Can you work these out from the drawing? Everything is in mm from the part's minimum corner. Coordinates: 2 decimals unless noted, no trailing zeros. Loops run counter-clockwise (first coordinate to the right, second up) from the corner with the lowest first, then second, coordinate; pieces in that order, holes last.
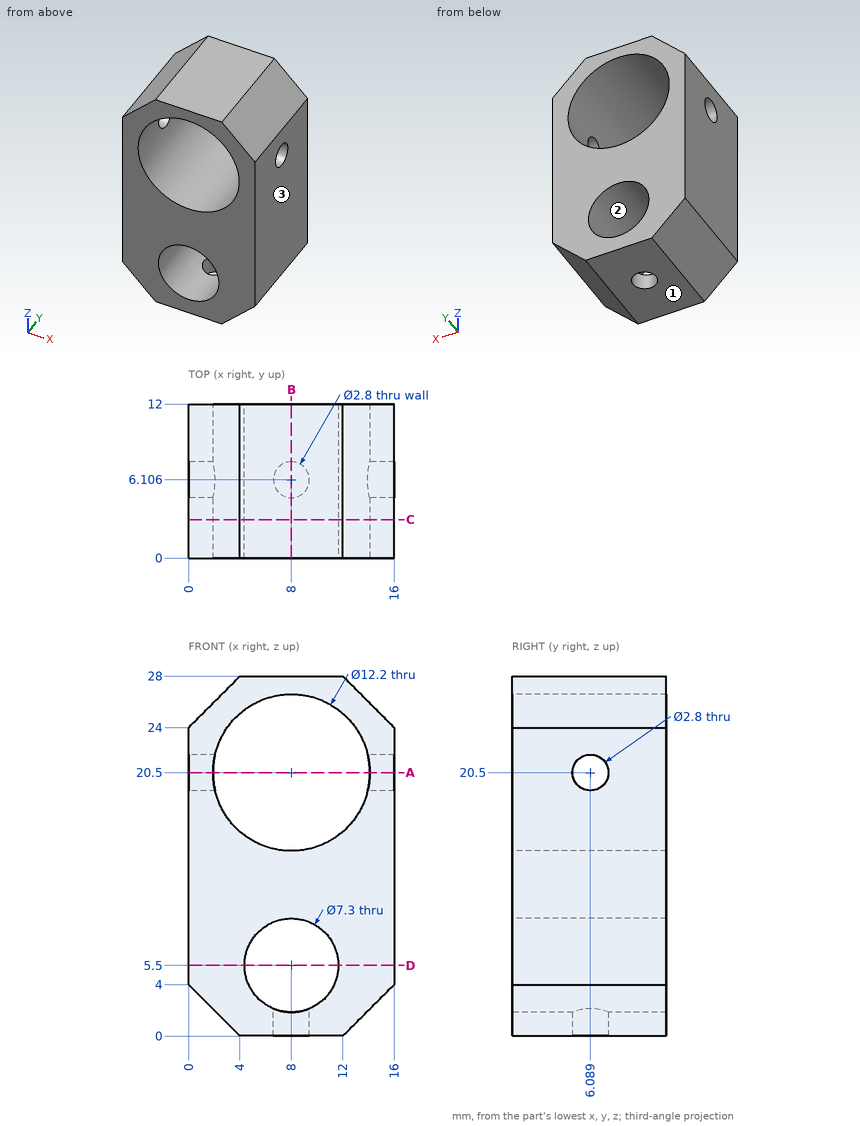
1) If I drill on L1, parallel to Z at x = 8, y = 9.75; L2, parallel to Z at x = 8, y = 6.75; L3, parallel to X at y = 1, z = 17, over which ranges is the centre line in solid material (lowest first)?
2) Imagine slicing it at B-B on x = 8. List the corners of the cut face in (y, z) for me.
3) Imagine slicing it at D-D on z = 5.5. List the corners of the cut face in (x, y) for me, plus the area to 3 significant figures.
4) Imagine slicing it at C-C on y = 3. List the corners of the cut face in (x, z) for me.
5) Will these pins go through, and if not, where does the flat tip stop? pin 1 (2.5 mm diameter, centred on y = 6.09, z = 20.5, fed in from +X); pin 2 (1 mm diameter, centred on x = 2, y = 7, fed in from -Z).
6) Imagine slicing it at A-A on z = 20.5. List the corners of the cut face in (x, y) for me.
7) We'd pull the mould along X, two halves only. Please class the marked faces 1, 2 and 3: released by +X, released by -X, zero draft, split by the parting line, or undercut.
Solved:
1. L1: z = 0 to 1.85, 9.15 to 14.4, 26.6 to 28
1. L2: z = 9.15 to 14.4, 26.6 to 28
1. L3: x = 0 to 3, 13 to 16
2. outline: (0, 0) - (4.71, 0) - (4.71, 1.85) - (0, 1.85) - close; (0, 9.15) - (12, 9.15) - (12, 14.4) - (0, 14.4) - close; (0, 26.6) - (12, 26.6) - (12, 28) - (0, 28) - close; (7.51, 0) - (12, 0) - (12, 1.85) - (7.51, 1.85) - close
3. outline: (0, 0) - (4.35, 0) - (4.35, 12) - (0, 12) - close; (11.65, 0) - (16, 0) - (16, 12) - (11.65, 12) - close
3. area: 104 mm2
4. outline: (0, 4) - (4, 0) - (12, 0) - (16, 4) - (16, 24) - (12, 28) - (4, 28) - (0, 24) - close; hole circle Ø12.2 at (8, 20.5); hole circle Ø7.3 at (8, 5.5)
5. pin 1: passes through
5. pin 2: stops at z = 1.5
6. outline: (0, 0) - (1.9, 0) - (1.9, 4.69) - (0, 4.69) - close; (0, 7.49) - (1.9, 7.49) - (1.9, 12) - (0, 12) - close; (14.1, 0) - (16, 0) - (16, 4.69) - (14.1, 4.69) - close; (14.1, 7.49) - (16, 7.49) - (16, 12) - (14.1, 12) - close
7. face 1: zero draft
7. face 2: undercut
7. face 3: released by +X
